from build123d import *

# Parameters (mm, degrees)
SKETCH1_R                                           = 47.5
SKETCH1_R_2                                         = 35
BOSS_EXTRUDE1_DEPTH                                 = 7
SKETCH2_R                                           = 2.25
SKETCH2_R_2                                         = 1.75
CUT_EXTRUDE1_DEPTH                                  = 68.538877693
CSK_FOR_M4_COUNTERSUNK_FLAT_HEAD_SCREW1_D           = 4.5
CSK_FOR_M4_COUNTERSUNK_FLAT_HEAD_SCREW1_CSINK_D     = 9.4
CSK_FOR_M4_COUNTERSUNK_FLAT_HEAD_SCREW1_CSINK_ANGLE = 90
BOSS_EXTRUDE2_START                                 = -7
SKETCH4_R                                           = 35
BOSS_EXTRUDE2_DEPTH                                 = 7
SKETCH6_R                                           = 1.75
CUT_EXTRUDE2_DEPTH                                  = 30
SKETCH2_2_R                                         = 2.25
SKETCH2_2_R_2                                       = 1.75
CUT_EXTRUDE3_DEPTH                                  = 68.538877693


# Read off the part's stored shape, not the designer's step: CSK for M4 Countersunk Flat Head Screw2
with BuildPart() as part:
    # Sketch1 → Boss-Extrude1 (new body)
    with BuildSketch(Plane(origin=(0, 0, 0), x_dir=(1, 0, 0), z_dir=(0, 1, 0))):
        with Locations(Location((0, 0, 0), (0, 0, 270))):
            Circle(SKETCH1_R)
        with Locations(Location((0, 0, 0), (0, 0, 270))):
            Circle(SKETCH1_R_2, mode=Mode.SUBTRACT)
    extrude(amount=BOSS_EXTRUDE1_DEPTH)

    # Sketch2 → Cut-Extrude1 (cut, through all)
    with BuildSketch(Plane(origin=(0, 7, 0), x_dir=(1, 0, 0), z_dir=(0, 1, 0))):
        with Locations(Location((0, 41.25, 0), (0, 0, 270))):
            Circle(SKETCH2_R)
        with Locations(Location((41.25, 0, 0), (0, 0, 270))):
            Circle(SKETCH2_R)
        with Locations(Location((0, -41.25, 0), (0, 0, 90))):
            Circle(SKETCH2_R)
        with Locations(Location((-41.25, 0, 0), (0, 0, 90))):
            Circle(SKETCH2_R)
        with Locations((0, 25)):
            Circle(SKETCH2_R_2)
        with Locations((25, 0)):
            Circle(SKETCH2_R_2)
        with Locations((0, -25)):
            Circle(SKETCH2_R_2)
        with Locations((-25, 0)):
            Circle(SKETCH2_R_2)
    extrude(amount=-CUT_EXTRUDE1_DEPTH, mode=Mode.SUBTRACT)

    # CSK for M4 Countersunk Flat Head Screw1 (through all)
    with Locations(Plane(origin=(0, 7, 41.25), x_dir=(0, 0, 1), z_dir=(0, 1, 0))):
        with Locations((0, 0), (-41.25, 41.25), (-82.5, 0), (-41.25, -41.25)):
            CounterSinkHole(CSK_FOR_M4_COUNTERSUNK_FLAT_HEAD_SCREW1_D / 2, CSK_FOR_M4_COUNTERSUNK_FLAT_HEAD_SCREW1_CSINK_D / 2, counter_sink_angle=CSK_FOR_M4_COUNTERSUNK_FLAT_HEAD_SCREW1_CSINK_ANGLE)

    # Sketch4 → Boss-Extrude2 (add)
    with BuildSketch(Plane(origin=(0, 7, 0), x_dir=(1, 0, 0), z_dir=(0, 1, 0)).offset(BOSS_EXTRUDE2_START)):
        Circle(SKETCH4_R)
    extrude(amount=BOSS_EXTRUDE2_DEPTH)

    # Sketch6 → Cut-Extrude2 (cut)
    with BuildSketch(Plane(origin=(0, 7, 0), x_dir=(1, 0, 0), z_dir=(0, 1, 0))):
        with Locations(Location((0, 0, 0), (0, 0, 270))):
            Circle(SKETCH6_R)
    extrude(amount=-CUT_EXTRUDE2_DEPTH, mode=Mode.SUBTRACT)

    # Sketch2<2> → Cut-Extrude3 (cut, through all)
    with BuildSketch(Plane(origin=(0, 7, 0), x_dir=(1, 0, 0), z_dir=(0, 1, 0))):
        with Locations(Location((0, 41.25, 0), (0, 0, 270))):
            Circle(SKETCH2_2_R)
        with Locations(Location((41.25, 0, 0), (0, 0, 270))):
            Circle(SKETCH2_2_R)
        with Locations(Location((0, -41.25, 0), (0, 0, 270))):
            Circle(SKETCH2_2_R)
        with Locations(Location((-41.25, 0, 0), (0, 0, 270))):
            Circle(SKETCH2_2_R)
        with Locations(Location((0, 25, 0), (0, 0, 270))):
            Circle(SKETCH2_2_R_2)
        with Locations(Location((25, 0, 0), (0, 0, 270))):
            Circle(SKETCH2_2_R_2)
        with Locations(Location((0, -25, 0), (0, 0, 270))):
            Circle(SKETCH2_2_R_2)
        with Locations(Location((-25, 0, 0), (0, 0, 270))):
            Circle(SKETCH2_2_R_2)
    extrude(amount=-CUT_EXTRUDE3_DEPTH, mode=Mode.SUBTRACT)

    # CSK for M4 Countersunk Flat Head Scr 2 → CSK for M4 Countersunk Flat Head Screw2 (revolve, cut)
    with BuildSketch(Plane.XY.offset(-25)):
        Polygon((1.75, 0), (4.7, 0), (2.25, 2.45), (2.25, 4.55), (4.7, 7), (1.75, 7), align=None)
    revolve(axis=Axis((0, 0, -25), (0, 1, 0)), mode=Mode.SUBTRACT)

    # CSK for M4 Countersunk Flat Head Scr 3 o → CSK for M4 Countersunk Flat Head Scr 3 (revolve, cut)
    with BuildSketch(Plane(origin=(25, 0, 0), x_dir=(1, 0, 0), z_dir=(0, 0, 1))):
        Polygon((1.75, 0), (2.25, 0), (2.25, 4.55), (4.7, 7), (1.75, 7), align=None)
    revolve(axis=Axis((25, 0, 0), (0, 1, 0)), mode=Mode.SUBTRACT)

    # CSK for M4 Countersunk Flat Head Scr 4 o → CSK for M4 Countersunk Flat Head Scr 4 (revolve, cut)
    with BuildSketch(Plane.XY.offset(25)):
        Polygon((1.75, 0), (2.25, 0), (2.25, 4.55), (4.7, 7), (1.75, 7), align=None)
    revolve(axis=Axis((0, 0, 25), (0, 1, 0)), mode=Mode.SUBTRACT)

    # CSK for M4 Countersunk Flat Head Scr 5 o → CSK for M4 Countersunk Flat Head Scr 5 (revolve, cut)
    with BuildSketch(Plane(origin=(-25, 0, 0), x_dir=(1, 0, 0), z_dir=(0, 0, 1))):
        Polygon((1.75, 0), (2.25, 0), (2.25, 4.55), (4.7, 7), (1.75, 7), align=None)
    revolve(axis=Axis((-25, 0, 0), (0, 1, 0)), mode=Mode.SUBTRACT)


solid = part.part
Build history of the part. All positions in model axes, mm. Round coordinates to 2 decimals unless told otherwise and drop trailing zeros. Write each loop counter-clockwise with the first axis right and the second up, starting at its lowest first coordinate (ties: lowest second). Pieces come first, ordered by that corner, then holes. Notation, with made-up numbers: (3, 10) - (47, 10) arc R20 cw to (47, 33) - close; hole circle Ø1 at (-14, 82.25). An arc over 180 degrees is marked (long way). One line per question, with ' | ' between items.
1. Band-saw the part on B-B, the plane x = -25. Write the cut outline in (y, z), and give its area (3 significant figures).
Results are:
outline: (0, -40.39) - (7, -40.39) - (7, -4.7) - (4.55, -2.25) - (0, -2.25) - close; (0, 2.25) - (4.55, 2.25) - (7, 4.7) - (7, 40.39) - (0, 40.39) - close | area: 528 mm^2
2. Band-saw the part on C-C, the plane z = 25. Write the cut outline in (x, y), and give its area (3 significant figures).
Results are:
outline: (-40.39, 0) - (-2.25, 0) - (-2.25, 4.55) - (-4.7, 7) - (-40.39, 7) - close; (2.25, 0) - (40.39, 0) - (40.39, 7) - (4.7, 7) - (2.25, 4.55) - close | area: 528 mm^2
3. Drop flat-ended pins along their axis: pin 1 Ø7 at (x, z) = (41.25, 0) entering from -Y; pin 2 Ø2 at (y, z) = (6, 14) entering from -X; pin 3 Ø4 at (x, y) = (10.5, 1) entering from -Z; pin 4 Ø3.5 at (x, z) = (-25, 0) entering from -Y. Give the stop position or say it passes through.
Results are:
pin 1: y = 0 | pin 2: x = -45.69 | pin 3: z = -46.73 | pin 4: through
4. Band-saw the part on D-D, the plane x = 8.5. Write the cut outline in (y, z), and give its area (3 significant figures).
Results are:
outline: (0, -46.73) - (7, -46.73) - (7, 46.73) - (0, 46.73) - close | area: 654 mm^2
5. Band-saw the part on A-A, the plane z = -25. Write the cut outline in (x, y), and give its area (3 significant figures).
Results are:
outline: (-40.39, 0) - (-4.7, 0) - (-2.25, 2.45) - (-2.25, 4.55) - (-4.7, 7) - (-40.39, 7) - close; (2.25, 2.45) - (4.7, 0) - (40.39, 0) - (40.39, 7) - (4.7, 7) - (2.25, 4.55) - close | area: 522 mm^2
6. Mould opens along X. For faces 1 (the face through (1, 7, 10)), 2 (the face through (-43.48, 2.31, 0.29)), 3 (the face through (-46.37, 3.45, -10.3)) say: released by +X, released by -X, zero draft, split by the parting line, or undercut.
Results are:
face 1: zero draft | face 2: undercut | face 3: split by the parting line
7. Drill centre lines: line 1 along X through (y, z) = (1.1, 0); line 2 along X through (y, z) = (1.65, -41.25); line 3 along X through (y, z) = (5.25, -19). Where is each one in solid material? Low to high. Write a range as from..to.
Results are:
line 1: -47.5..-43.5, -39..-27.25, -22.75..-1.75, 1.75..22.75, 27.25..39, 43.5..47.5 | line 2: -23.55..-2.25, 2.25..23.55 | line 3: -43.53..43.53
